Autodesk Inventor part; units mm, degrees
ref_plane "YZ Plane" through (0, 0, 0) normal (1, 0, 0) x (0, 1, 0)
ref_plane "XZ Plane" through (0, 0, 0) normal (0, 1, 0) x (-1, 0, 0)
ref_plane "XY Plane" through (0, 0, 0) normal (0, 0, 1) x (1, 0, 0)
sketch "Sketch1" plane through (0, 0, 0) normal (0, 0, 1) x (1, 0, 0)
  arc A0 (60, 0) -> (-60, 0) centre (0, -84.947) ccw
  line L0 (60, 0) -> (60, 30)
  line L1 (60, 30) -> (60, 35)
  line L2 (-60, 35) -> (-60, 0)
  line L3 (60, 35) -> (-60, 35)
  point P0 (0, 0)
  dimension "d2" = 104
  dimension "d9" = 30
  dimension "d10" = 5
extrude "Extrusion1" add sketch "Sketch1" along normal blind 180
fillet "Fillet5" radius 5 2 edges at (-60, 35, 90) (60, 35, 90)
sketch "Sketch5" plane through (-55, 35, 0) normal (0, 1, 0) x (1, 0, 0)
  line L0 (115, -180) -> (-5, -180)
  circle A0 centre (55, -160) radius 1.25
  circle A1 centre (55, -20) radius 1.25
  point P0 (55, 0)
extrude "Extrusion5" cut sketch "Sketch5" against normal blind 3
thread "Thread4"
thread "Thread5"
properties part number "NEW Dudukan di Bearring"
Read the model definition and answer for the solid it produces. Units are mm, in the model's axes. Give positions to 0.01 mm unless a question says otherwise; leave off trailing zeros. Write each loop counter-clockwise with the first axis right and the second up, starting at its lowest first coordinate (ties: lowest second). Pieces come first, ordered by that corner, then holes. Notation, with made-up numbers: (56, -1) - (71, -1) arc R20 cw to (71, 18) - close; hole circle Ø8 at (29, 43.5). An arc over 180 degrees is marked (long way). Answer in a Markdown table with one row per item. Add a question column.
Item 1: Section A-A, the plane z = 42.5 is taken. Write down the section's boundary in (x, y), and give its area (3 significant figures).
Item 2: Flat-ended cylindrical pins translate along their axes: P1, Ø5, axis at x = -21, z = 40, coming from the -Y side; P2, Ø4, axis at x = 0, z = 20, coming from the -Y side. Find the tip coordinate at first contact, or state that the pin passes through.
Item 3: Determine the mould class of faces 1 (the face through (-58, 34, 91)), 2 (the face through (-0.9, 19.05, 88.74)), 3 (the face through (1, 35, 89)) for opening direction X: pulls with the +X half, pulls with the -X half, needs draft (parallel to the pull), parting line crosses it, or undercut.
Item 4: Find the intervals of material crossed by L1, parallel to Z at x = 0, y = 34; L2, parallel to X at y = 7.5, z = 138.5; L3, parallel to X at y = 33.35, z = 160, in increasing order.
Item 5: Section B-B, the plane x = 50 is taken. Write down the section's boundary in (y, z).
Item 6: Section C-C, the plane x = -5.5 is taken. Write down the section's boundary in (y, z), and give its area (3 significant figures).
Recorded:
| question | item | result |
|---|---|---|
| 1 | outline | (-60, 0) arc R104 cw to (60, 0) - (60, 30) arc R5 ccw to (55, 35) - (-55, 35) arc R5 ccw to (-60, 30) - close |
| 1 | area | 2,630 mm2 |
| 2 | P1 | stops at y = 16.36 |
| 2 | P2 | stops at y = 19.03 |
| 3 | face 1 | pulls with the -X half |
| 3 | face 2 | undercut |
| 3 | face 3 | needs draft |
| 4 | L1 | z = 0 to 18.75, 21.25 to 158.75, 161.25 to 180 |
| 4 | L2 | x = -60 to -47.64, 47.64 to 60 |
| 4 | L3 | x = -58.71 to -1.25, 1.25 to 58.71 |
| 5 | outline | (6.25, 0) - (35, 0) - (35, 180) - (6.25, 180) - close |
| 6 | outline | (18.91, 0) - (35, 0) - (35, 180) - (18.91, 180) - close |
| 6 | area | 2,900 mm2 |
